Part model, mm, in its own coordinate system. Face numbers are marked on the shaded views. Coordinates: 2 decimals unless noted, no trailing zeros. Write each loop counter-clockwise with the first axis right and the second up, starting at its lowest first coordinate (ties: lowest second). Pieces come first, ordered by that corner, then holes. Notation, with made-up numbers: (-38.75, -3.75) -> (-15.75, -3.75) arc R8 ccw to (-15.75, 4.25) -> close; hole circle Ø7 at (-17, 33.5). An arc over 180 degrees is marked (long way). Write item = value, one per line. Start each with the question number.
Q1. Pin check, flat tips, straight feed: P1, Ø3, axis at y = -12.7, z = 0, coming from the -X side; P2, Ø5, axis at x = 17.5, z = -3.5, coming from the -Y side; P3, Ø1.5, axis at x = 23.5, z = 3.5, coming from the +Y side. Stop position of each tip, or through.
Q2. Band-saw the part on A-A, the plane x = -7. List the corners of the cut face in (y, z).
Q3. Band-saw the part on D-D, the plane x = 22. List the corners of the cut face in (y, z), plus the area to 3 significant figures.
Q4. Band-saw the part on C-C, the plane x = 5. List the corners of the cut face in (y, z).
Q5. Pull direction X, two halves, no side cores. Call the marked faces 1, 2 and 3: released by +X, released by -X, zero draft, split by the parting line, or undercut.
Q6. Band-saw the part on B-B, the plane y = 0. List the corners of the cut face in (x, z).
Q7. Probe line 1 (Y direction, x = -7, z = 0); line 2 (Z direction, x = -7.5, y = 0); line 3 (Y direction, x = -7, z = -1.5). List the from-to ranges inside material, lowest first.
Autodesk Inventor part; units mm, degrees
ref_plane "YZ Plane" through (0, 0, 0) normal (1, 0, 0) x (0, 1, 0)
ref_plane "XZ Plane" through (0, 0, 0) normal (0, 1, 0) x (-1, 0, 0)
ref_plane "XY Plane" through (0, 0, 0) normal (0, 0, 1) x (1, 0, 0)
sketch "Sketch2" plane through (0, 0, 0) normal (0, 0, 1) x (1, 0, 0)
  line L0 (-12.7, 19.05) -> (12.7, 19.05)
  line L1 (12.7, 19.05) -> (12.7, -19.05) construction
  line L2 (12.7, -19.05) -> (-12.7, -19.05)
  line L3 (-12.7, -19.05) -> (-12.7, 19.05)
  line L4 (-12.7, 19.05) -> (12.7, -19.05) construction
  line L5 (12.7, 19.05) -> (-12.7, -19.05) construction
  arc A0 (12.7, -19.05) -> (12.7, 19.05) centre (12.7, 0) ccw
  point P0 (0, 0)
  point P1 (31.75, 0)
  dimension "d0" = 38.1
  dimension "d1" = 25.4
  dimension "d4" = 44.45
extrude "Extrusion1" add sketch "Sketch2" along normal mid plane 9.525
sketch "Sketch3" plane through (0, 0, -4.7625) normal (0, 0, -1) x (-1, 0, 0)
  arc A0 (-12.7, 19.05) -> (-12.7, -19.05) centre (-12.7, 0) ccw construction
  point P0 (0, 0)
hole "Hole1" at (12.7, 0, -4.7625) direction (0, 0, 1) diameter 28.575 end through all
sketch "Sketch4" plane through (-12.7, -19.05, 4.7625) normal (-1, 0, 0) x (0, 0, 1)
  line L0 (-4.7625, 6.35) -> (-4.7625, 31.75) construction
  point P0 (-4.7625, 19.05)
  point P1 (-4.7625, 19.05)
  dimension "d12" = 25.4
hole "Hole2" at (-12.7, -12.7, 0) at (-12.7, 12.7, 0) at (-12.7, 0, 0) direction (1, 0, 0) diameter 3.9624 depth 13.6144 tip angle 118
properties part number "PLATE,BEARING,DRIVE,ELEVATOR" material "Aluminum, 7075-T6"
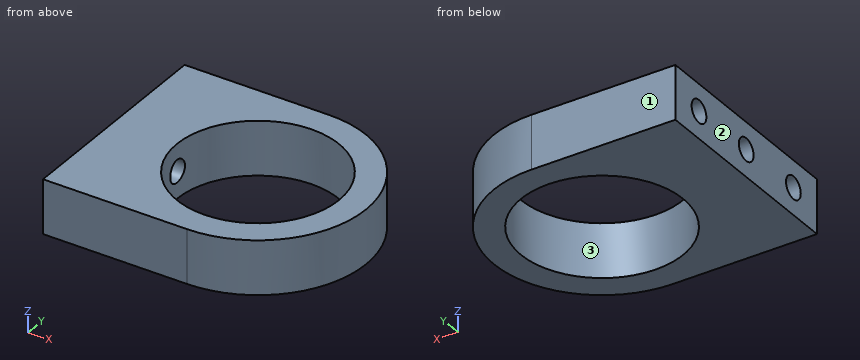
Ans:
q1.P1 = 1.2
q1.P2 = -18.91
q1.P3 = 16.18
q2.outline = (-19.05, -4.76) -> (19.05, -4.76) -> (19.05, 4.76) -> (-19.05, 4.76) -> close; hole circle Ø3.96 at (-12.7, 0); hole circle Ø3.96 at (0, 0); hole circle Ø3.96 at (12.7, 0)
q3.outline = (-16.63, -4.76) -> (-10.85, -4.76) -> (-10.85, 4.76) -> (-16.63, 4.76) -> close; (10.85, -4.76) -> (16.63, -4.76) -> (16.63, 4.76) -> (10.85, 4.76) -> close
q3.area = 110 mm2
q4.outline = (-19.05, -4.76) -> (-12.04, -4.76) -> (-12.04, 4.76) -> (-19.05, 4.76) -> close; (12.04, -4.76) -> (19.05, -4.76) -> (19.05, 4.76) -> (12.04, 4.76) -> close
q5.face_1 = zero draft
q5.face_2 = released by -X
q5.face_3 = undercut
q6.outline = (-12.7, -4.76) -> (-1.59, -4.76) -> (-1.59, -1.98) -> (-12.7, -1.98) -> close; (-12.7, 1.98) -> (-1.59, 1.98) -> (-1.59, 4.76) -> (-12.7, 4.76) -> close; (26.99, -4.76) -> (31.75, -4.76) -> (31.75, 4.76) -> (26.99, 4.76) -> close
q7.line_1 = -19.05 to -14.68, -10.72 to -1.98, 1.98 to 10.72, 14.68 to 19.05
q7.line_2 = -4.76 to -1.98, 1.98 to 4.76
q7.line_3 = -19.05 to -13.99, -11.41 to -1.29, 1.29 to 11.41, 13.99 to 19.05
